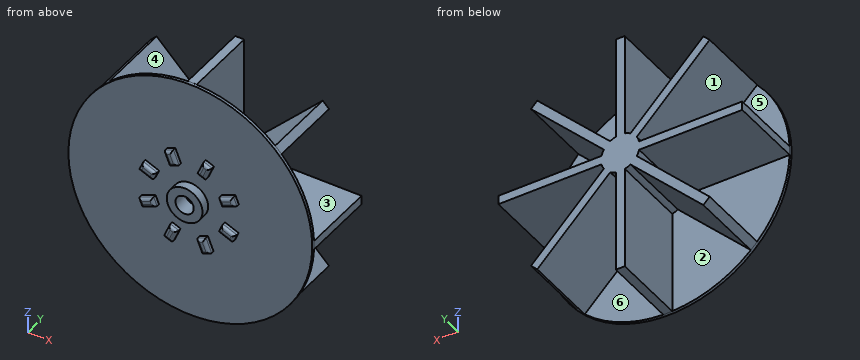
from build123d import *

# Parameters (mm, degrees)
SKETCH1_R            = 41
BOSS_EXTRUDE1_DEPTH  = 1
SKETCH6_W            = 3
SKETCH6_H            = 41
BOSS_EXTRUDE7_DEPTH  = 25
SKETCH7_R            = 6
BOSS_EXTRUDE8_DEPTH  = 24
SKETCH9_R            = 6
CUT_EXTRUDE3_DEPTH   = 5
CIRPATTERN1_COUNT    = 8
SKETCH11_R           = 6
CUT_EXTRUDE5_DEPTH   = 6
BOSS_EXTRUDE9_DEPTH  = 2
CIRPATTERN2_COUNT    = 8
FILLET1_R            = 1
SKETCH13_R           = 6.5
BOSS_EXTRUDE17_DEPTH = 6
SKETCH16_R           = 6.5
SKETCH16_R_2         = 6
BOSS_EXTRUDE18_DEPTH = 25
SKETCH15_R           = 6
BOSS_EXTRUDE19_DEPTH = 3
SKETCH17_R           = 3.075
CUT_EXTRUDE10_DEPTH  = 5


with BuildPart() as part:
    # Sketch1 → Boss-Extrude1 (new body)
    with BuildSketch(Plane(origin=(0, 0, 0), x_dir=(1, 0, 0), z_dir=(0, 1, 0))):
        Circle(SKETCH1_R)
    extrude(amount=BOSS_EXTRUDE1_DEPTH)

    # Sketch6 → Boss-Extrude7 (add)
    with BuildSketch(Plane(origin=(0, 1, 0), x_dir=(1, 0, 0), z_dir=(0, 1, 0))):
        with Locations((0, -20.5)):
            Rectangle(SKETCH6_W, SKETCH6_H)
    boss_extrude7 = extrude(amount=BOSS_EXTRUDE7_DEPTH)

    # Sketch7 → Boss-Extrude8 (add)
    with BuildSketch(Plane.XZ):
        Circle(SKETCH7_R)
    extrude(amount=-BOSS_EXTRUDE8_DEPTH)

    # Sketch9 → Cut-Extrude3 (cut)
    with BuildSketch(Plane(origin=(0, 26, 0), x_dir=(1, 0, 0), z_dir=(0, 1, 0))):
        Circle(SKETCH9_R)
    extrude(amount=-CUT_EXTRUDE3_DEPTH, mode=Mode.SUBTRACT)

    # CirPattern1: Boss-Extrude7 ×8 about axis
    cirpattern1_axis = Axis((0, 0, 0), (0, 1, 0))
    for i in range(1, CIRPATTERN1_COUNT):
        add(boss_extrude7.rotate(cirpattern1_axis, i * 360 / CIRPATTERN1_COUNT))

    # Sketch11 → Cut-Extrude5 (cut)
    with BuildSketch(Plane(origin=(0, 26, 0), x_dir=(1, 0, 0), z_dir=(0, 1, 0))):
        Circle(SKETCH11_R)
    extrude(amount=-CUT_EXTRUDE5_DEPTH, mode=Mode.SUBTRACT)

    # Sketch10 → Boss-Extrude9 (add)
    with BuildSketch(Plane(origin=(0, 0, 0), x_dir=(-1, 0, 0), z_dir=(0, -1, 0))):
        Polygon((-3.142992858, 11.677824964), (-5.920826915, 10.544847493), (-7.809122701, 15.174570921), (-5.031288644, 16.307548393), align=None)
    boss_extrude9 = extrude(amount=BOSS_EXTRUDE9_DEPTH)

    # CirPattern2: Boss-Extrude9 ×8 about axis
    cirpattern2_axis = Axis((0, 0, 0), (0, 1, 0))
    for i in range(1, CIRPATTERN2_COUNT):
        add(boss_extrude9.rotate(cirpattern2_axis, i * 360 / CIRPATTERN2_COUNT))

    # Fillet1
    fillet1_edges = [part.edges().sort_by_distance(p)[0] for p in [
        (4.087140751, -2, -13.992686678),
        (6.420205673, -2, -15.741059657),
        (6.864974808, -2, -12.859709207),
        (4.531909887, -2, -11.111336228),
        (-7.004278697, -2, -12.784368578),
        (-6.590839059, -2, -15.670380994),
        (-4.238917345, -2, -13.947457824),
        (-4.652356983, -2, -11.061445408),
        (-13.992686678, -2, -4.087140751),
        (-15.741059657, -2, -6.420205673),
        (-12.859709207, -2, -6.864974808),
        (-11.111336228, -2, -4.531909887),
        (-12.784368578, -2, 7.004278697),
        (-15.670380994, -2, 6.590839059),
        (-13.947457824, -2, 4.238917345),
        (-11.061445408, -2, 4.652356983),
        (-4.087140751, -2, 13.992686678),
        (-6.420205673, -2, 15.741059657),
        (-6.864974808, -2, 12.859709207),
        (-4.531909887, -2, 11.111336228),
        (7.004278697, -2, 12.784368578),
        (6.590839059, -2, 15.670380994),
        (4.238917345, -2, 13.947457824),
        (4.652356983, -2, 11.061445408),
        (13.992686678, -2, 4.087140751),
        (15.741059657, -2, 6.420205673),
        (12.859709207, -2, 6.864974808),
        (11.111336228, -2, 4.531909887),
        (12.784368578, -2, -7.004278697),
        (15.670380994, -2, -6.590839059),
        (13.947457824, -2, -4.238917345),
        (11.061445408, -2, -4.652356983),
    ]]
    fillet(fillet1_edges, radius=FILLET1_R)

    # Sketch13 → Boss-Extrude17 (add)
    with BuildSketch(Plane(origin=(0, 20, 0), x_dir=(1, 0, 0), z_dir=(0, 1, 0))):
        Circle(SKETCH13_R)
    extrude(amount=BOSS_EXTRUDE17_DEPTH)

    # Sketch16 → Boss-Extrude18 (add)
    with BuildSketch(Plane(origin=(0, 26, 0), x_dir=(1, 0, 0), z_dir=(0, 1, 0))):
        Circle(SKETCH16_R)
        Circle(SKETCH16_R_2, mode=Mode.SUBTRACT)
    extrude(amount=-BOSS_EXTRUDE18_DEPTH)

    # Sketch15 → Boss-Extrude19 (add)
    with BuildSketch(Plane.XZ):
        Circle(SKETCH15_R)
    extrude(amount=BOSS_EXTRUDE19_DEPTH)

    # Sketch17 → Cut-Extrude10 (cut)
    with BuildSketch(Plane.XZ.offset(3)):
        Circle(SKETCH17_R)
    extrude(amount=-CUT_EXTRUDE10_DEPTH, mode=Mode.SUBTRACT)


solid = part.part
Work out the finished part from the listing and answer in its coordinate system (mm). Face numbers are marked on the shaded views. A direction names the side the tool comes from. Coordinates: 2 decimals unless noted, no trailing zeros. Order: outer loops, then holes, each group sorted by start corner. A loop starts at its lowest first (then second) coordinate and runs counter-clockwise, first axis right, second up. Notation, with made-up numbers: (18.5, -22.75) - (75.5, -22.75) arc R21 cw to (75.5, 15.25) - close; hole circle Ø7 at (17.25, -4). An arc over 180 degrees is marked (long way). Put each result on its own line as item: value. Start each with the question number.
1) Find the intervals of material crossed by line 1 (Z direction, x = -28, y = 24.75); line 2 (Z direction, x = 12, y = 5.75); line 3 (X direction, y = 8.75, z = -13), in increasing order. Write a range as from..to.
2) Find section C-C (x = 24). Give the vertices of the cut face in (y, z), plus the area to 3 significant figures.
3) Find section B-B (x = -24.5). Give the vertices of the cut face in (y, z).
4) Flat-ended cylindrical pins translate along their axes: pin 1 (7.5 mm diameter, centred on y = 12.5, z = -17, fed in from +X); pin 2 (13 mm diameter, centred on x = 28, z = -11, fed in from +Y); pin 3 (0.6 mm diameter, centred on x = 13, z = -6, fed in from -Y). Find the tip coordinate at first contact, or state that the pin passes through.
5) For a pull along X with two mould halves and no side action, classify the marked faces 1, 2 and 3 as released by +X, released by -X, zero draft, split by the parting line, or undercut.
6) For the marked faces 4, 5 and 6, determine the directions among +Z, -Z, +X, -X, +Y, -Y from which every point of the face is accessible in a straight line to the end or side of a thin tool.
Results list:
1. line 1: z = -29.98..-25.88, -1.5..1.5, 25.88..29.98
1. line 2: z = -14.12..-9.88, -1.5..1.5, 9.88..14.12
1. line 3: x = -15.12..-10.88, -1.5..1.5, 10.88..15.12
2. outline: (0, -33.24) - (1, -33.24) - (1, -26.12) - (26, -26.12) - (26, -21.88) - (1, -21.88) - (1, -1.5) - (26, -1.5) - (26, 1.5) - (1, 1.5) - (1, 21.88) - (26, 21.88) - (26, 26.12) - (1, 26.12) - (1, 33.24) - (0, 33.24) - close
2. area: 354 mm^2
3. outline: (0, -32.87) - (1, -32.87) - (1, -26.62) - (26, -26.62) - (26, -22.38) - (1, -22.38) - (1, -1.5) - (26, -1.5) - (26, 1.5) - (1, 1.5) - (1, 22.38) - (26, 22.38) - (26, 26.62) - (1, 26.62) - (1, 32.87) - (0, 32.87) - close
4. pin 1: stops at x = 22.87
4. pin 2: stops at y = 1
4. pin 3: stops at y = -2
5. face 1: released by -X
5. face 2: undercut
5. face 3: zero draft
6. face 4: +Z, +Y
6. face 5: -X, +Y
6. face 6: -Z, +Y
